Geometry check sheet. Reference: drawing and pictorial views, mm from the part's lowest x, y, z. A direction names the side the tool comes from. Round coordinates to 2 decimals unless told otherwise and drop trailing zeros. Order: outer loops, then holes, each group sorted by start corner. A loop starts at its lowest first (then second) coordinate and runs counter-clockwise, first axis right, second up.
(1) Draft check along Z on the marked faces 1, 2 and 3. Enter one of: pulls with the +Z half, pulls with the -Z half, needs draft (parallel to the pull), parting line crosses it, or undercut.
(2) Cross-section at D-D on z = 4. Enter the section's corners in (x, y).
(3) Cross-section at C-C on y = 19. Enter the section's corners in (x, z).
(4) Set-up check for the marked faces 4, 5, 6, 7 and 8: record each of +Z, -Z, +X, -X, +Y, -Y from which the full face is reachable in a straight line by a thin tool's end or side.
(5) Gauge pin test, flat ends, axial feed: P1, Ø4, axis at x = 106.5, z = 17.5, coming from the +Y side; P2, Ø8.5, axis at x = 56, z = 13.5, coming from the +Y side; P3, Ø2, axis at x = 18.5, y = 21.5, coming from the +Z side. Record the tip position at first contact, or that the pin passes through.
(6) Cross-section at A-A on z = 41. Enter the section's corners in (x, y).
(7) Cross-section at B-B on x = 63.5. Enter the section's corners in (y, z), and give its area (3 significant figures).
(8) Thickness scan on L1, parallel to Z at x = 63.5, y = 38; L2, parallel to X at y = 23.5, z = 24; L3, parallel to X at y = 15.5, z = 18.5 (1 decimal). Record the ranges inside material, lowest first.
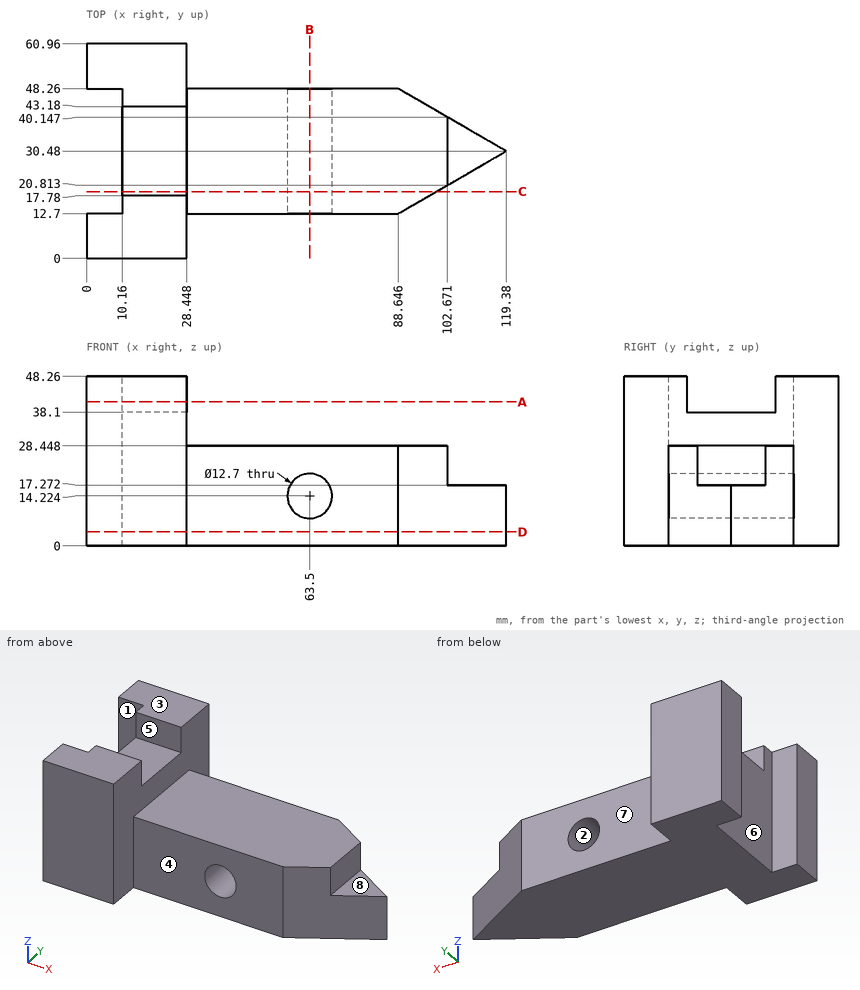
Found:
1. face 1: needs draft
1. face 2: undercut
1. face 3: pulls with the +Z half
2. outline: (0, 0) - (28.45, 0) - (28.45, 12.7) - (88.65, 12.7) - (119.38, 30.48) - (88.65, 48.26) - (28.45, 48.26) - (28.45, 60.96) - (0, 60.96) - (0, 48.26) - (10.16, 48.26) - (10.16, 12.7) - (0, 12.7) - close
3. outline: (10.16, 0) - (99.54, 0) - (99.54, 28.45) - (28.45, 28.45) - (28.45, 38.1) - (10.16, 38.1) - close; hole circle Ø12.7 at (63.5, 14.22)
4. face 4: +Z, -Z, +X, -Y
4. face 5: +Z, +X, -X
4. face 6: +Z, -Z, -X
4. face 7: +Z, -Z, +X, +Y
4. face 8: +Z, +X, +Y, -Y
5. P1: stops at y = 39.08
5. P2: stops at y = 48.26
5. P3: stops at z = 38.1
6. outline: (0, 0) - (28.45, 0) - (28.45, 17.78) - (10.16, 17.78) - (10.16, 12.7) - (0, 12.7) - close; (0, 48.26) - (10.16, 48.26) - (10.16, 43.18) - (28.45, 43.18) - (28.45, 60.96) - (0, 60.96) - close
7. outline: (12.7, 0) - (48.26, 0) - (48.26, 7.87) - (12.7, 7.87) - close; (12.7, 20.57) - (48.26, 20.57) - (48.26, 28.45) - (12.7, 28.45) - close
7. area: 560 mm2
8. L1: z = 0 to 7.87, 20.57 to 28.45
8. L2: x = 10.16 to 102.67
8. L3: x = 10.2 to 58.8, 68.2 to 93.5
